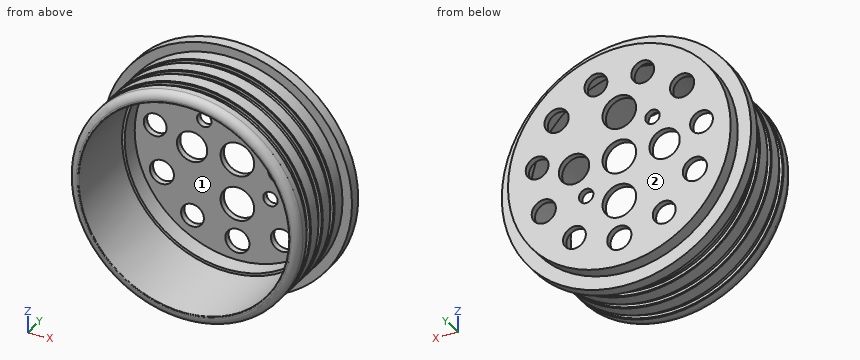
```python
from build123d import *

# Parameters (mm, degrees)
CHAMFER1_SIZE      = 0.5
FILLET3_R          = 5
FILLET4_R          = 0.5
CUT_EXTRUDE1_REACH = 70.81
SKETCH3_R          = 11.125
SKETCH3_R_2        = 10.05
SKETCH3_R_3        = 8
SKETCH3_R_4        = 7.55
SKETCH3_R_5        = 4.7625
SKETCH4_R          = 68
CUT_EXTRUDE2_DEPTH = 12.06


with BuildPart() as part:
    # Sketch2 → Revolve1 (revolve)
    with BuildSketch(Plane.XY):
        Polygon((76.25, 52.75), (76.25, 42.75), (73.75, 42.75), (73.75, 38.5), (76.25, 38.5), (76.25, 28.5), (73.75, 28.5), (73.75, 24.25), (76.25, 24.25), (76.25, 14.25), (73.75, 14.25), (73.75, 10), (76.25, 10), (76.25, 0), (69.75, 0), (69.75, 52.75), (0, 52.75), (0, 60.25), (0, 68.810209945), (73.75, 68.810209945), (73.75, 60.25), (82.55, 60.25), (82.55, 52.75), align=None)
    revolve(axis=Axis((0, 0, 0), (0, 1, 0)))

    # Chamfer1
    chamfer1_edges = [part.edges().sort_by_distance(p)[0] for p in [
        (-76.25, 42.75, 0),
        (-76.25, 38.5, 0),
        (-76.25, 28.5, 0),
        (-76.25, 24.25, 0),
        (-76.25, 14.25, 0),
        (-76.25, 10, 0),
    ]]
    chamfer(chamfer1_edges, length=CHAMFER1_SIZE)

    # Fillet3
    fillet3_edges = [part.edges().sort_by_distance(p)[0] for p in [
        (-76.25, 0, 0),
    ]]
    fillet(fillet3_edges, radius=FILLET3_R)

    # Fillet4
    fillet4_edges = [part.edges().sort_by_distance(p)[0] for p in [
        (-69.75, 0, 0),
    ]]
    fillet(fillet4_edges, radius=FILLET4_R)

    # Sketch3 → Cut-Extrude1 (cut, up to next)
    with BuildSketch(Plane(origin=(0, 68.810209945, 0), x_dir=(1, 0, 0), z_dir=(0, 1, 0)), mode=Mode.PRIVATE) as cut_extrude1_sk1:
        Circle(SKETCH3_R)
    cut_extrude1_tool1 = extrude(cut_extrude1_sk1.sketch, amount=-CUT_EXTRUDE1_REACH, mode=Mode.PRIVATE) & part.part
    add(cut_extrude1_tool1.solids().sort_by_distance((0, 68.81021, 0))[0], mode=Mode.SUBTRACT)
    # Sketch3 → Cut-Extrude1 (cut, up to next)
    with BuildSketch(Plane(origin=(0, 68.810209945, 0), x_dir=(1, 0, 0), z_dir=(0, 1, 0)), mode=Mode.PRIVATE) as cut_extrude1_sk2:
        with Locations((30, 0)):
            Circle(SKETCH3_R_2)
    cut_extrude1_tool2 = extrude(cut_extrude1_sk2.sketch, amount=-CUT_EXTRUDE1_REACH, mode=Mode.PRIVATE) & part.part
    add(cut_extrude1_tool2.solids().sort_by_distance((30, 68.81021, 0))[0], mode=Mode.SUBTRACT)
    # Sketch3 → Cut-Extrude1 (cut, up to next)
    with BuildSketch(Plane(origin=(0, 68.810209945, 0), x_dir=(1, 0, 0), z_dir=(0, 1, 0)), mode=Mode.PRIVATE) as cut_extrude1_sk3:
        with Locations((0, -30)):
            Circle(SKETCH3_R)
    cut_extrude1_tool3 = extrude(cut_extrude1_sk3.sketch, amount=-CUT_EXTRUDE1_REACH, mode=Mode.PRIVATE) & part.part
    add(cut_extrude1_tool3.solids().sort_by_distance((0, 68.81021, 30))[0], mode=Mode.SUBTRACT)
    # Sketch3 → Cut-Extrude1 (cut, up to next)
    with BuildSketch(Plane(origin=(0, 68.810209945, 0), x_dir=(1, 0, 0), z_dir=(0, 1, 0)), mode=Mode.PRIVATE) as cut_extrude1_sk4:
        with Locations((-30, 0)):
            Circle(SKETCH3_R_2)
    cut_extrude1_tool4 = extrude(cut_extrude1_sk4.sketch, amount=-CUT_EXTRUDE1_REACH, mode=Mode.PRIVATE) & part.part
    add(cut_extrude1_tool4.solids().sort_by_distance((-30, 68.81021, 0))[0], mode=Mode.SUBTRACT)
    # Sketch3 → Cut-Extrude1 (cut, up to next)
    with BuildSketch(Plane(origin=(0, 68.810209945, 0), x_dir=(1, 0, 0), z_dir=(0, 1, 0)), mode=Mode.PRIVATE) as cut_extrude1_sk5:
        with Locations((0, 30)):
            Circle(SKETCH3_R)
    cut_extrude1_tool5 = extrude(cut_extrude1_sk5.sketch, amount=-CUT_EXTRUDE1_REACH, mode=Mode.PRIVATE) & part.part
    add(cut_extrude1_tool5.solids().sort_by_distance((0, 68.81021, -30))[0], mode=Mode.SUBTRACT)
    # Sketch3 → Cut-Extrude1 (cut, up to next)
    with BuildSketch(Plane(origin=(0, 68.810209945, 0), x_dir=(1, 0, 0), z_dir=(0, 1, 0)), mode=Mode.PRIVATE) as cut_extrude1_sk6:
        with Locations((0, 55)):
            Circle(SKETCH3_R_3)
    cut_extrude1_tool6 = extrude(cut_extrude1_sk6.sketch, amount=-CUT_EXTRUDE1_REACH, mode=Mode.PRIVATE) & part.part
    add(cut_extrude1_tool6.solids().sort_by_distance((0, 68.81021, -55))[0], mode=Mode.SUBTRACT)
    # Sketch3 → Cut-Extrude1 (cut, up to next)
    with BuildSketch(Plane(origin=(0, 68.810209945, 0), x_dir=(1, 0, 0), z_dir=(0, 1, 0)), mode=Mode.PRIVATE) as cut_extrude1_sk7:
        with Locations((29.73524496, 46.268944306)):
            Circle(SKETCH3_R_4)
    cut_extrude1_tool7 = extrude(cut_extrude1_sk7.sketch, amount=-CUT_EXTRUDE1_REACH, mode=Mode.PRIVATE) & part.part
    add(cut_extrude1_tool7.solids().sort_by_distance((29.735245, 68.81021, -46.268944))[0], mode=Mode.SUBTRACT)
    # Sketch3 → Cut-Extrude1 (cut, up to next)
    with BuildSketch(Plane(origin=(0, 68.810209945, 0), x_dir=(1, 0, 0), z_dir=(0, 1, 0)), mode=Mode.PRIVATE) as cut_extrude1_sk8:
        with Locations((50.029759744, 22.847825715)):
            Circle(SKETCH3_R_3)
    cut_extrude1_tool8 = extrude(cut_extrude1_sk8.sketch, amount=-CUT_EXTRUDE1_REACH, mode=Mode.PRIVATE) & part.part
    add(cut_extrude1_tool8.solids().sort_by_distance((50.02976, 68.81021, -22.847826))[0], mode=Mode.SUBTRACT)
    # Sketch3 → Cut-Extrude1 (cut, up to next)
    with BuildSketch(Plane(origin=(0, 68.810209945, 0), x_dir=(1, 0, 0), z_dir=(0, 1, 0)), mode=Mode.PRIVATE) as cut_extrude1_sk9:
        with Locations((54.440179303, -7.827316105)):
            Circle(SKETCH3_R_4)
    cut_extrude1_tool9 = extrude(cut_extrude1_sk9.sketch, amount=-CUT_EXTRUDE1_REACH, mode=Mode.PRIVATE) & part.part
    add(cut_extrude1_tool9.solids().sort_by_distance((54.440179, 68.81021, 7.827316))[0], mode=Mode.SUBTRACT)
    # Sketch3 → Cut-Extrude1 (cut, up to next)
    with BuildSketch(Plane(origin=(0, 68.810209945, 0), x_dir=(1, 0, 0), z_dir=(0, 1, 0)), mode=Mode.PRIVATE) as cut_extrude1_sk10:
        with Locations((41.566226589, -36.017340367)):
            Circle(SKETCH3_R_3)
    cut_extrude1_tool10 = extrude(cut_extrude1_sk10.sketch, amount=-CUT_EXTRUDE1_REACH, mode=Mode.PRIVATE) & part.part
    add(cut_extrude1_tool10.solids().sort_by_distance((41.566227, 68.81021, 36.01734))[0], mode=Mode.SUBTRACT)
    # Sketch3 → Cut-Extrude1 (cut, up to next)
    with BuildSketch(Plane(origin=(0, 68.810209945, 0), x_dir=(1, 0, 0), z_dir=(0, 1, 0)), mode=Mode.PRIVATE) as cut_extrude1_sk11:
        with Locations((15.495290626, -52.772113549)):
            Circle(SKETCH3_R_4)
    cut_extrude1_tool11 = extrude(cut_extrude1_sk11.sketch, amount=-CUT_EXTRUDE1_REACH, mode=Mode.PRIVATE) & part.part
    add(cut_extrude1_tool11.solids().sort_by_distance((15.495291, 68.81021, 52.772114))[0], mode=Mode.SUBTRACT)
    # Sketch3 → Cut-Extrude1 (cut, up to next)
    with BuildSketch(Plane(origin=(0, 68.810209945, 0), x_dir=(1, 0, 0), z_dir=(0, 1, 0)), mode=Mode.PRIVATE) as cut_extrude1_sk12:
        with Locations((-15.495290626, -52.772113549)):
            Circle(SKETCH3_R_4)
    cut_extrude1_tool12 = extrude(cut_extrude1_sk12.sketch, amount=-CUT_EXTRUDE1_REACH, mode=Mode.PRIVATE) & part.part
    add(cut_extrude1_tool12.solids().sort_by_distance((-15.495291, 68.81021, 52.772114))[0], mode=Mode.SUBTRACT)
    # Sketch3 → Cut-Extrude1 (cut, up to next)
    with BuildSketch(Plane(origin=(0, 68.810209945, 0), x_dir=(1, 0, 0), z_dir=(0, 1, 0)), mode=Mode.PRIVATE) as cut_extrude1_sk13:
        with Locations((-41.566226589, -36.017340367)):
            Circle(SKETCH3_R_3)
    cut_extrude1_tool13 = extrude(cut_extrude1_sk13.sketch, amount=-CUT_EXTRUDE1_REACH, mode=Mode.PRIVATE) & part.part
    add(cut_extrude1_tool13.solids().sort_by_distance((-41.566227, 68.81021, 36.01734))[0], mode=Mode.SUBTRACT)
    # Sketch3 → Cut-Extrude1 (cut, up to next)
    with BuildSketch(Plane(origin=(0, 68.810209945, 0), x_dir=(1, 0, 0), z_dir=(0, 1, 0)), mode=Mode.PRIVATE) as cut_extrude1_sk14:
        with Locations((-54.440179303, -7.827316105)):
            Circle(SKETCH3_R_4)
    cut_extrude1_tool14 = extrude(cut_extrude1_sk14.sketch, amount=-CUT_EXTRUDE1_REACH, mode=Mode.PRIVATE) & part.part
    add(cut_extrude1_tool14.solids().sort_by_distance((-54.440179, 68.81021, 7.827316))[0], mode=Mode.SUBTRACT)
    # Sketch3 → Cut-Extrude1 (cut, up to next)
    with BuildSketch(Plane(origin=(0, 68.810209945, 0), x_dir=(1, 0, 0), z_dir=(0, 1, 0)), mode=Mode.PRIVATE) as cut_extrude1_sk15:
        with Locations((-50.029759744, 22.847825715)):
            Circle(SKETCH3_R_3)
    cut_extrude1_tool15 = extrude(cut_extrude1_sk15.sketch, amount=-CUT_EXTRUDE1_REACH, mode=Mode.PRIVATE) & part.part
    add(cut_extrude1_tool15.solids().sort_by_distance((-50.02976, 68.81021, -22.847826))[0], mode=Mode.SUBTRACT)
    # Sketch3 → Cut-Extrude1 (cut, up to next)
    with BuildSketch(Plane(origin=(0, 68.810209945, 0), x_dir=(1, 0, 0), z_dir=(0, 1, 0)), mode=Mode.PRIVATE) as cut_extrude1_sk16:
        with Locations((-29.73524496, 46.268944306)):
            Circle(SKETCH3_R_4)
    cut_extrude1_tool16 = extrude(cut_extrude1_sk16.sketch, amount=-CUT_EXTRUDE1_REACH, mode=Mode.PRIVATE) & part.part
    add(cut_extrude1_tool16.solids().sort_by_distance((-29.735245, 68.81021, -46.268944))[0], mode=Mode.SUBTRACT)
    # Sketch3 → Cut-Extrude1 (cut, up to next)
    with BuildSketch(Plane(origin=(0, 68.810209945, 0), x_dir=(1, 0, 0), z_dir=(0, 1, 0)), mode=Mode.PRIVATE) as cut_extrude1_sk17:
        with Locations((21.940611049, 20.459950802)):
            Circle(SKETCH3_R_5)
    cut_extrude1_tool17 = extrude(cut_extrude1_sk17.sketch, amount=-CUT_EXTRUDE1_REACH, mode=Mode.PRIVATE) & part.part
    add(cut_extrude1_tool17.solids().sort_by_distance((21.940611, 68.81021, -20.459951))[0], mode=Mode.SUBTRACT)
    # Sketch3 → Cut-Extrude1 (cut, up to next)
    with BuildSketch(Plane(origin=(0, 68.810209945, 0), x_dir=(1, 0, 0), z_dir=(0, 1, 0)), mode=Mode.PRIVATE) as cut_extrude1_sk18:
        with Locations((-21.940611049, -20.459950802)):
            Circle(SKETCH3_R_5)
    cut_extrude1_tool18 = extrude(cut_extrude1_sk18.sketch, amount=-CUT_EXTRUDE1_REACH, mode=Mode.PRIVATE) & part.part
    add(cut_extrude1_tool18.solids().sort_by_distance((-21.940611, 68.81021, 20.459951))[0], mode=Mode.SUBTRACT)

    # Sketch4 → Cut-Extrude2 (cut)
    with BuildSketch(Plane.XZ.offset(-52.75)):
        Circle(SKETCH4_R)
    extrude(amount=-CUT_EXTRUDE2_DEPTH, mode=Mode.SUBTRACT)


solid = part.part
```
Input: part model. Units: mm. Frame: model coordinates. Face numbers are marked on the shaded views. Coordinates: 2 decimals unless noted, no trailing zeros. Write each loop counter-clockwise with the first axis right and the second up, starting at its lowest first coordinate (ties: lowest second). Pieces come first, ordered by that corner, then holes.
1) Section A-A on y = 56. Output: boundary loops of the cut face in (x, z), and give its area (3 significant figures).
2) Material intervals for line 1 along Z through (x, y) = (0, 67.55) (3 decimals); line 2 along Y through (x, z) = (69, 29); line 3 along X through (y, z) = (21, 0), sorted ascending.
3) Mould query, pull axis X, two halves, no side actions, for the marked faces 1 and 2. Classes: pulls with the +X half, pulls with the -X half, needs draft (parallel to the pull), parting line crosses it, or undercut.
4) Pin query (flat end, axial travel): pin 1 Ø9 at (x, z) = (-15.5, 52.77) entering from -Y; pin 2 Ø10 at (x, y) = (-29.5, 22) entering from +Z; pin 3 Ø2 at (x, y) = (49.5, 32) entering from +Z; pin 4 Ø1 at (x, z) = (-51, 31) entering from -Y. Return the tip coordinate at first contact, or that it passes through.
5) Section B-B on z = -7.5. State how many separate pieces and enclosed holes the cut face has, and give its area (3 significant figures).
Check result:
1. outline: circle Ø165.1 at (0, 0); hole circle Ø136 at (0, 0)
1. area: 6,880 mm2
2. line 1: z = -73.75 to -63, -47 to -41.125, -18.875 to -11.125, 11.125 to 18.875, 41.125 to 73.75
2. line 2: y = 1.53 to 10, 14.25 to 24.25, 28.5 to 38.5, 42.75 to 60.25
2. line 3: x = -76.25 to -69.75, 69.75 to 76.25
3. face 1: undercut
3. face 2: needs draft
4. pin 1: passes through
4. pin 2: stops at z = 72.21
4. pin 3: stops at z = 58.84
4. pin 4: stops at y = 64.81
5. separate pieces: 4
5. enclosed holes: 0
5. area: 1,300 mm2
